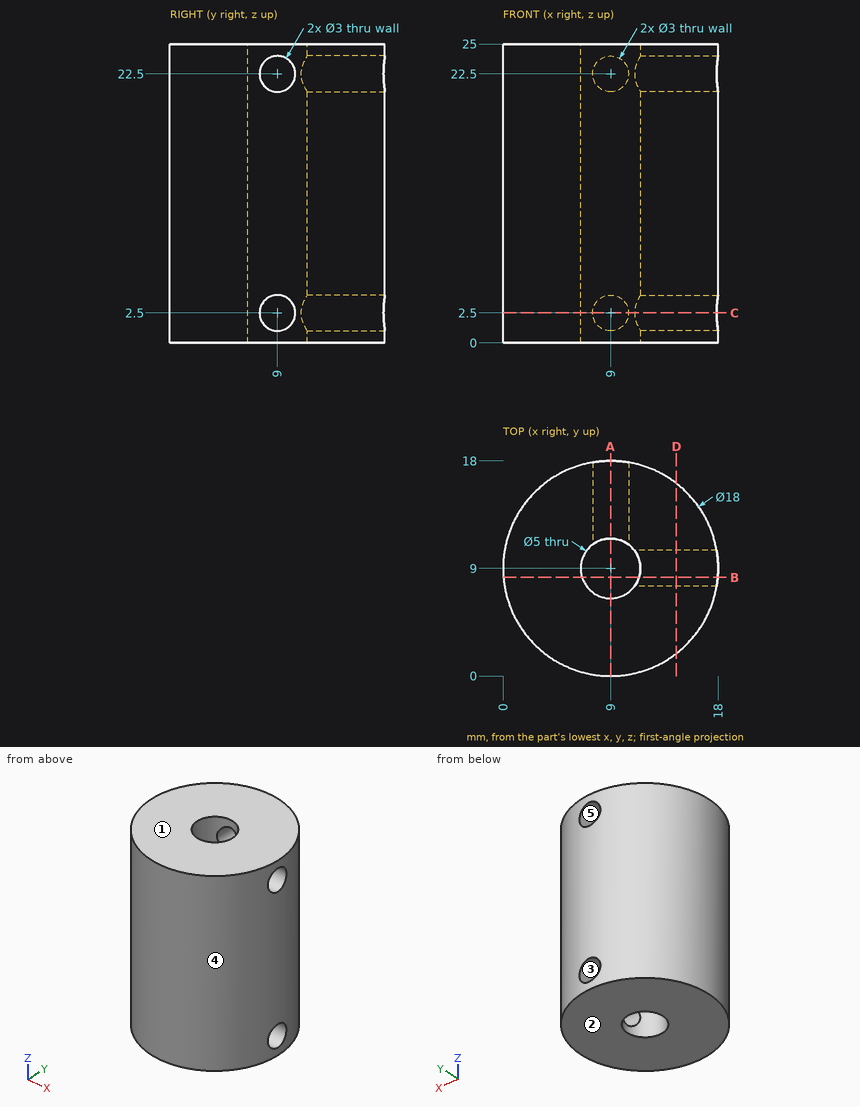
Answer from the drawing. Dimensions are ordinates in mm from the lowest x, y and z of the part. A direction names the side the tool comes from. Round coordinates to 2 decimals unless told otherwise and drop trailing zeros. Write each loop counter-clockwise with the first axis right and the second up, starting at its lowest first coordinate (ties: lowest second). Pieces come first, ordered by that corner, then holes. Notation, with made-up numbers: M 69.25,-10 L 93.25,-10 A29 ccw 93.25,11 Z; hole C 21.5,-30 d11. An arc over 180 degrees is marked long. Write each question's results on one line, items separated by ' | '. Start each with the question number.
Item 1: Find section C-C on z = 2.5. Write down the section's boundary in (x, y), and give its area (3 significant figures).
Item 2: Find section B-B on y = 8.25. Write down the section's boundary in (x, z), and give its area (3 significant figures).
Item 3: Which of the six approach directions +Z, -Z, +X, -X, +Y, -Y give full straight-line access (tool end or side, diameter ignored) to the marked faces 4 and 5?
Item 4: The mould has two halves that part along Z. Classify the marked faces 1, 2 and 3: +Z half, -Z half, draft (parallel to the pull), parting line (faces both ways), or undercut.
Item 5: Find section A-A on x = 9. Write down the section's boundary in (y, z).
Item 6: Given pin 1 Ø4 at (x, z) = (13, 21) entering from +Y; pin 2 Ø2.5 at (y, z) = (9, 2.5) entering from +X; pin 3 Ø1.8 at (x, z) = (9, 22.5) entering from +Y, each flat-ended and moving along its own axis, determine where each tip first touches the part or whether it passes through.
Item 7: Find section D-D on x = 14.5. Write down the section's boundary in (y, z).
Item 8: Straight lines are drawn through the part: probe 1 along Y at (x, z) = (9, 6.5); probe 2 along Z at (x, y) = (8.75, 15.5); probe 3 along Y at (x, z) = (14.75, 2.5). For each, find the intervals that lie inside material, in ascending order.
Answer block:
1) outline: M 7.5,11 L 7.5,17.87 A9 ccw long 17.87,7.5 L 11,7.5 A2.5 cw long Z; M 10.5,11 A2.5 cw 11,10.5 L 17.87,10.5 A9 ccw 10.5,17.87 Z | area: 195 mm²
2) outline: M 0.03,0 L 6.62,0 L 6.62,25 L 0.03,25 Z; M 11.38,0 L 17.97,0 L 17.97,1.2 L 11.38,1.2 Z; M 11.38,3.8 L 17.97,3.8 L 17.97,21.2 L 11.38,21.2 Z; M 11.38,23.8 L 17.97,23.8 L 17.97,25 L 11.38,25 Z | area: 295 mm²
3) face 4: +Z, -Z | face 5: +Y
4) face 1: +Z half | face 2: -Z half | face 3: undercut
5) outline: M 0,0 L 6.5,0 L 6.5,25 L 0,25 Z; M 11.5,0 L 18,0 L 18,1 L 11.5,1 Z; M 11.5,4 L 18,4 L 18,21 L 11.5,21 Z; M 11.5,24 L 18,24 L 18,25 L 11.5,25 Z
6) pin 1: stops at y = 17.77 | pin 2: stops at x = 6.83 | pin 3: stops at y = 6.67
7) outline: M 1.88,0 L 16.12,0 L 16.12,25 L 1.88,25 Z; hole C 9,2.5 d3; hole C 9,22.5 d3
8) probe 1: y = 0 to 6.5, 11.5 to 18 | probe 2: z = 0 to 1.02, 3.98 to 21.02, 23.98 to 25 | probe 3: y = 2.08 to 7.5, 10.5 to 15.92
